```python
from build123d import *

# Parameters (mm, degrees)
BOSS_EXTRUDE1_DEPTH = 76.99375
SKETCH2_R           = 3.4925
BOSS_EXTRUDE2_DEPTH = 1.5875


with BuildPart() as part:
    # Sketch1 → Boss-Extrude1 (new body, symmetric)
    with BuildSketch(Plane(origin=(0, 0, 0), x_dir=(0, 0, -1), z_dir=(1, 0, 0))):
        with BuildLine():
            ThreePointArc((-26.121491242, 15.08125), (7.806629448, 29.134737735), (30.1625, 0))
            Line((30.1625, 0), (31.75, 0))
            ThreePointArc((31.75, 0), (8.217504682, 30.668144985), (-27.49630657, 15.875))
            Line((-27.49630657, 15.875), (-26.121491242, 15.08125))
        make_face()
    extrude(amount=BOSS_EXTRUDE1_DEPTH, both=True)

    # Sketch2 → Boss-Extrude2 (add)
    with BuildSketch(Plane(origin=(76.99375, 0, 0), x_dir=(0, 0, -1), z_dir=(1, 0, 0))):
        with BuildLine():
            Line((-19.05, 0), (-3.4925, 0))
            ThreePointArc((-3.4925, 0), (0, 3.4925), (3.4925, 0))
            Line((3.4925, 0), (19.05, 0))
            ThreePointArc((19.05, 0), (25.4, -6.35), (31.75, 0))
            ThreePointArc((31.75, 0), (0, 31.75), (-31.75, 0))
            ThreePointArc((-31.75, 0), (-25.4, -6.35), (-19.05, 0))
        make_face()
        with Locations((-25.4, 0)):
            Circle(SKETCH2_R, mode=Mode.SUBTRACT)
        with Locations((25.4, 0)):
            Circle(SKETCH2_R, mode=Mode.SUBTRACT)
    boss_extrude2 = extrude(amount=BOSS_EXTRUDE2_DEPTH)

    # Mirror1: Boss-Extrude2 across plane
    add(boss_extrude2.mirror(Plane(origin=(0, 0, 0), x_dir=(0, 0, 1), z_dir=(1, 0, 0))))


solid = part.part
```
Could you check a few things on this model? Use its own coordinates, in mm. A direction names the side the tool comes from. Coordinates: 2 decimals unless noted, no trailing zeros. Write each loop counter-clockwise with the first axis right and the second up, starting at its lowest first coordinate (ties: lowest second). Pieces come first, ordered by that corner, then holes. Notation, with made-up numbers: M 86.25,44 L 145.25,44 A17 ccw 145.25,56 Z; hole C 35,60.25 d3. An arc over 180 degrees is marked long. Answer as CSV lines item,"result". Start each with the question number.
1) Please list where these lines run through material, in increasing order: line 1 (Y direction, x = -77.8, z = 25.4); line 2 (X direction, y = 26, z = -6.5); line 3 (Z direction, x = -0.5, y = 17). Write a range as from..to.
2) For faces 3 (the flat face through (76.994, 12, 0)), 4 (the cylindrical face through (-77.78, -6.35, -25.26)), which set-ups out of +Z, -Z, +X, -X, +Y, -Y let a thin tool reach every point of the face, with its end or its side?
3) For P1, Ø0.8, axis at x = 78, z = 13, coming from the -Y side; P2, Ø5, axis at x = -58.5, z = -15, coming from the +Y side; P3, Ø1.5, axis at x = 48.5, y = -0.5, coming from the +Z side; P4, Ø5.5, axis at y = 0, z = 25.4, coming from the +X side, each with a flat end and sliding along its axis, tell me the tip position at first contact or that it passes through.
4) I want a section at B-B, the plane y = 19.5. Please give me the cut outline in (x, z).
5) We'd pull the mould along Z, two halves only. Please class faces 1 (the flat face through (-78.581, 13, 0)), 2 (the flat face through (-76.994, 12, 0)): +Z half, -Z half, draft (parallel to the pull), parting line (faces both ways), or undercut.
6) I want a section at D-D, the plane y = 8. Please give me the cut outline in (x, z), and give its area (3 significant figures).
7) I want a section at A-A, the plane z = -25.4. Please give me the cut outline in (x, y).
8) I want a section at C-C, the plane z = 0. Please give me the cut outline in (x, y).
Data:
1,line 1,"y = -6.35..-3.49, 3.49..19.05"
1,line 2,"x = -78.58..-76.99, 76.99..78.58"
1,line 3,"z = -26.82..-24.92, 24.92..26.82"
2,face 3,"-Y"
2,face 4,"+X, -X, -Y"
3,P1,"stops at y = 0"
3,P2,"stops at y = 29.19"
3,P3,"stops at z = -30.16"
3,P4,"passes through"
4,outline,"M -78.58,-25.06 L 78.58,-25.06 L 78.58,25.06 L -78.58,25.06 Z; hole M -76.99,-23.01 L 76.99,-23.01 L 76.99,23.01 L -76.99,23.01 Z"
5,face 1,"draft"
5,face 2,"undercut"
6,outline,"M -78.58,-30.73 L 78.58,-30.73 L 78.58,30.73 L 76.99,30.73 L 76.99,-29.08 L -76.99,-29.08 L -76.99,30.73 L -78.58,30.73 Z"
6,area,"448 mm^2"
7,outline,"M -78.58,-6.35 L -76.99,-6.35 L -76.99,-3.49 L -78.58,-3.49 Z; M -78.58,3.49 L -76.99,3.49 L -76.99,16.27 L 76.99,16.27 L 76.99,3.49 L 78.58,3.49 L 78.58,19.05 L -78.58,19.05 Z; M 76.99,-6.35 L 78.58,-6.35 L 78.58,-3.49 L 76.99,-3.49 Z"
8,outline,"M -78.58,3.49 L -76.99,3.49 L -76.99,30.16 L 76.99,30.16 L 76.99,3.49 L 78.58,3.49 L 78.58,31.75 L -78.58,31.75 Z"
